from build123d import *

# Parameters (mm, degrees)
SKETCH_1_W          = 24
SKETCH_1_H          = 94
EXTRUDE_1_DEPTH     = 4
SKETCH_2_W          = 8
SKETCH_2_H          = 8
CUT_EXTRUDE_1_DEPTH = 5
SKETCH_3_W          = 8
SKETCH_3_H          = 8
CUT_EXTRUDE_2_DEPTH = 5
CUT_EXTRUDE_3_DEPTH = 0.5
CUT_EXTRUDE_4_DEPTH = 0.5
CUT_EXTRUDE_5_DEPTH = 0.5


with BuildPart() as part:
    # 草圖1 → 填料-伸長1 (new body)
    with BuildSketch(Plane(origin=(0, 4, 0), x_dir=(1, 0, 0), z_dir=(0, 1, 0))):
        Rectangle(SKETCH_1_W, SKETCH_1_H)
    extrude(amount=-EXTRUDE_1_DEPTH)

    # 草圖2 → 除料-伸長1 (cut, through all)
    with BuildSketch(Plane.XZ):
        with Locations((0, -43)):
            Rectangle(SKETCH_2_W, SKETCH_2_H)
    extrude(amount=-CUT_EXTRUDE_1_DEPTH, mode=Mode.SUBTRACT)

    # 草圖3 → 除料-伸長2 (cut, through all)
    with BuildSketch(Plane.XZ):
        with Locations((0, 43)):
            Rectangle(SKETCH_3_W, SKETCH_3_H)
    extrude(amount=-CUT_EXTRUDE_2_DEPTH, mode=Mode.SUBTRACT)

    # 草圖4 → 除料-伸長3 (cut)
    with BuildSketch(Plane(origin=(0, 4, 0), x_dir=(-1, 0, 0), z_dir=(0, 1, 0))):
        Polygon((-5.604611564, 15.070843631), (-5.604611564, 3.228998522), (3.921964275, 3.228998522), (3.921964275, 5.581554951), (-3.252055136, 5.581554951), (-3.252055136, 7.973642862), (1.530624471, 7.973642862), (1.530624471, 10.326199291), (-3.252055136, 10.326199291), (-3.252055136, 12.718289616), (3.921964275, 12.718289616), (3.921964275, 15.070843631), align=None)
    extrude(amount=-CUT_EXTRUDE_3_DEPTH, mode=Mode.SUBTRACT)

    # 草圖5 → 除料-伸長4 (cut)
    with BuildSketch(Plane(origin=(0, 4, 0), x_dir=(-1, 0, 0), z_dir=(0, 1, 0))):
        Polygon((1.512356153, -5.362438696), (1.512356153, -12.657328252), (-3.252055136, -12.657328252), (-3.252055136, -15.009884681), (3.864912581, -15.009884681), (3.864912581, -3.009884681), (-3.252055136, -3.009884681), (-3.252055136, -5.362438696), align=None)
    extrude(amount=-CUT_EXTRUDE_4_DEPTH, mode=Mode.SUBTRACT)

    # 草圖6 → 除料-伸長5 (cut)
    with BuildSketch(Plane(origin=(0, 4, 0), x_dir=(-1, 0, 0), z_dir=(0, 1, 0))):
        Polygon((-5.604611564, -12.657328252), (-3.262055136, -12.657328252), (-3.252055136, -5.372438696), (-5.604611564, -5.362438696), align=None)
    extrude(amount=-CUT_EXTRUDE_5_DEPTH, mode=Mode.SUBTRACT)


solid = part.part
Build history of the part. All positions in model axes, mm. A direction names the side the tool comes from. Round coordinates to 2 decimals unless told otherwise and drop trailing zeros. Write each loop counter-clockwise with the first axis right and the second up, starting at its lowest first coordinate (ties: lowest second). Pieces come first, ordered by that corner, then holes. Notation, with made-up numbers: M 64.25,52 L 112.25,52 A28 ccw 112.25,83 Z; hole C -6.5,-15 d1. An arc over 180 degrees is marked long. Answer as a JSON object with one key per item and string values. Group by question number.
(1) Which spindle directions (+Z, -Z, +X, -X, +Y, -Y) get a long thin tool onto all of the face, cutting with end or side? Do faces 4 (the flat face through (0, 2, 39)), 5 (the flat face through (4, 2, -43)), 6 (the flat face through (4, 3.5, -9)). Say none if no direction does.
(2) Flat gauge pins, fed straight in: pin 1 (10 mm diameter, centred on x = 5, z = -5.5, fed in from +Y); pin 2 (2 mm diameter, centred on x = 1, y = 1, fed in from +Z); pin 3 (0.6 mm diameter, centred on x = -1, y = 3.5, fed in from -Z). Where does each tip first touch, or does it go through?
(3) Cut at B-B (x = -0.5). Give the cut face in (y, z), and give its area (3 significant figures).
(4) Cut at C-C (y = 2.6). Give the cut face in (x, z).
(5) Drill centre lines: L1, parallel to Y at x = -3, z = -13.5; L2, parallel to Z at x = -2.25, y = 3.1. Where is each one in solid material? Low to high.
(6) Mould opens along X. For faces 1 (the flat face through (-4, 2, -43)), 2 (the flat face through (-12, 2, 1)), 3 (the flat face through (8, 2, 47)) say: pulls with the +X half, pulls with the -X half, needs draft (parallel to the pull), parting line crosses it, or undercut.
(7) Cut at A-A (z = 9). Give the cut face in (x, y).
Responses:
{
 "1": {"face 4": "+Z, +Y, -Y", "face 5": "-Z, +Y, -Y", "face 6": "+Y"},
 "2": {"pin 1": "stops at y = 4", "pin 2": "stops at z = 39", "pin 3": "stops at z = -39"},
 "3": {"outline": "M 0,-39 L 4,-39 L 4,-15.01 L 3.5,-15.01 L 3.5,-12.66 L 4,-12.66 L 4,-5.36 L 3.5,-5.36 L 3.5,-3.01 L 4,-3.01 L 4,3.23 L 3.5,3.23 L 3.5,5.58 L 4,5.58 L 4,7.97 L 3.5,7.97 L 3.5,10.33 L 4,10.33 L 4,12.72 L 3.5,12.72 L 3.5,15.07 L 4,15.07 L 4,39 L 0,39 Z", "area": "306 mm2"},
 "4": {"outline": "M -12,-47 L -4,-47 L -4,-39 L 4,-39 L 4,-47 L 12,-47 L 12,47 L 4,47 L 4,39 L -4,39 L -4,47 L -12,47 Z"},
 "5": {"L1": "y = 0 to 3.5", "L2": "z = -39 to 39"},
 "6": {"face 1": "undercut", "face 2": "pulls with the -X half", "face 3": "needs draft"},
 "7": {"outline": "M -12,0 L 12,0 L 12,4 L 5.6,4 L 5.6,3.5 L -1.53,3.5 L -1.53,4 L -12,4 Z"}
}
